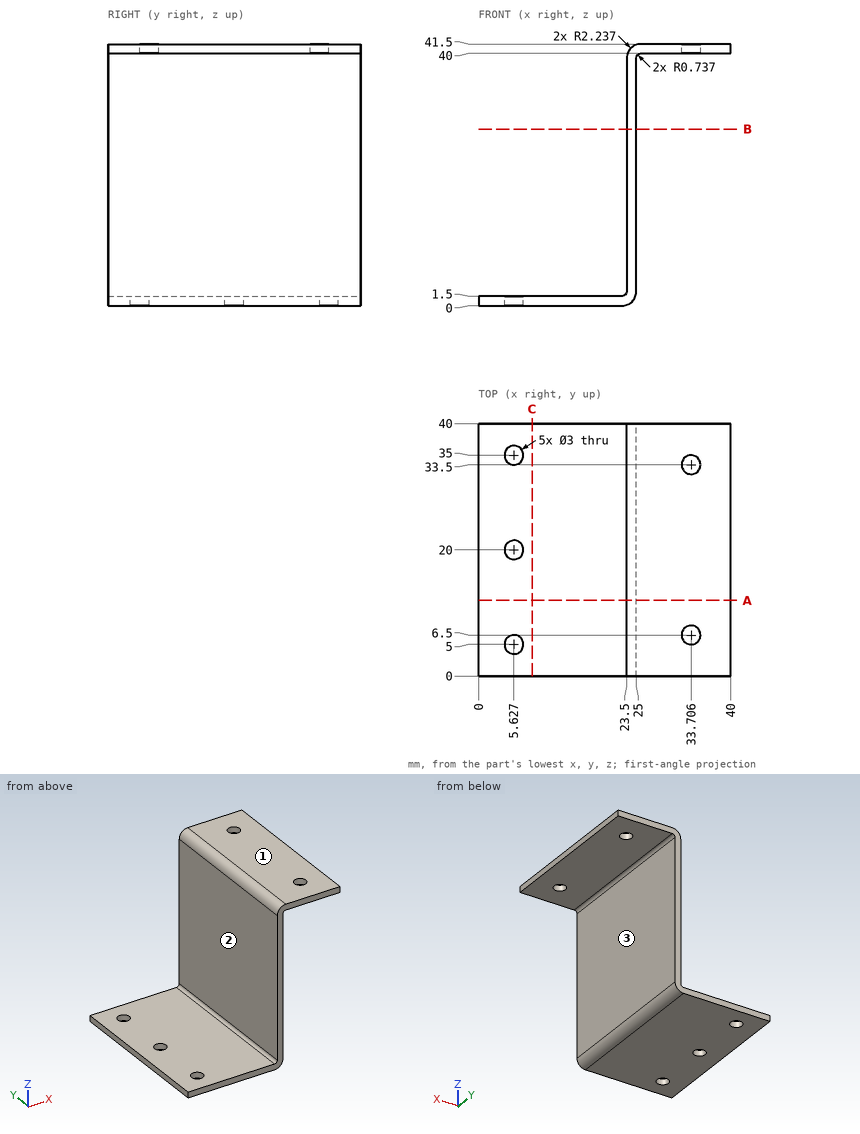
Here's the drawing with two shaded views (mm, measured from the low corner). I have some questions. A direction names the side the tool comes from. Give positions to 0.01 mm unless a question says otherwise; leave off trailing zeros. Loops run counter-clockwise (first coordinate to the right, second up) from the corner with the lowest first, then second, coordinate; pieces in that order, holes last. Notation, with made-up numbers: (41, 28) -> (86, 28) arc R23 cw to (86, 65) -> close; hole circle Ø1 at (40.25, 16). An arc over 180 degrees is marked (long way). One line per item, written item: value.
Q1. If I drill on line 1 along Z through (x, y) = (36, 32.5); line 2 along Z through (x, y) = (16, 20); line 3 along X through (y, z) = (34.5, 38.5), over which ranges is the centre line in solid material (lowest first)?
Answers follow:
line 1: 40 to 41.5
line 2: 0 to 1.5
line 3: 23.5 to 25
Q2. Suppose I cut it at C-C on x = 8.5. Please give me the cut outline in (y, z).
Answers follow:
outline: (0, 0) -> (40, 0) -> (40, 1.5) -> (0, 1.5) -> close
Q3. On a 3-axis mill with a long thin cutter (end or side, diameter ignored), from which of +Z, -Z, +X, -X, +Y, -Y can I reach the whole of each face in a straight line? I mean the marked faces 1, 2 and 3. Say none if no direction works.
Answers follow:
face 1: +Z, +X, -X, +Y, -Y
face 2: +Z, -X, +Y, -Y
face 3: -Z, +X, +Y, -Y
Q4. Suppose I cut it at A-A on y = 12. Please give me the cut outline in (x, z).
Answers follow:
outline: (0, 0) -> (22.76, 0) arc R2.24 ccw to (25, 2.24) -> (25, 39.26) arc R0.74 cw to (25.74, 40) -> (40, 40) -> (40, 41.5) -> (25.74, 41.5) arc R2.24 ccw to (23.5, 39.26) -> (23.5, 2.24) arc R0.74 cw to (22.76, 1.5) -> (0, 1.5) -> close
Q5. I'm going to push flat-ended pins straight in: pin 1 Ø12 at (y, z) = (8, 19) entering from -X; pin 2 Ø4 at (y, z) = (32.5, 30.5) entering from +X; pin 3 Ø18 at (x, y) = (12.5, 25.5) entering from +Z; pin 4 Ø2.5 at (x, y) = (5.63, 20) entering from +Z. Where does each tip first touch, or does it pass through?
Answers follow:
pin 1: x = 23.5
pin 2: x = 25
pin 3: z = 1.5
pin 4: through
Q6. Suppose I cut it at B-B on z = 28. Please give me the cut outline in (x, y).
Answers follow:
outline: (23.5, 0) -> (25, 0) -> (25, 40) -> (23.5, 40) -> close
